Read the model definition and answer for the solid it produces. Units are mm, in the model's axes. A direction names the side the tool comes from. Coordinates: 2 decimals unless noted, no trailing zeros. Loops run counter-clockwise (first coordinate to the right, second up) from the corner with the lowest first, then second, coordinate; pieces in that order, holes last. Notation, with made-up numbers: (-25.75, 24) -> (-11.75, 24) arc R33 cw to (-11.75, 52) -> close; hole circle Ø2 at (43, -3). An arc over 180 degrees is marked (long way). Answer as a JSON object with one key per item and string values. Group by question number.
1) Section C-C, the plane x = 35.5 is taken. Give the vertices of the cut face in (y, z), plus the area to 3 significant figures.
2) Flat-ended cylindrical pins translate along their axes: P1, Ø0.7, axis at x = 14.5, y = -2, coming from the -Z side; P2, Ø1.5, axis at y = -2, z = -1, coming from the -X side; P3, Ø10, axis at x = 8.5, z = 47, coming from the +Y side; P4, Ø0.5, axis at x = 24.5, y = -1, coming from the +Z side. Find the tip coordinate at first contact, or state that the pin passes through.
3) Consider probe 1 along Z at (x, y) = (-2, -2.45); probe 2 along X at (y, z) = (-2.5, 113); probe 3 along Z at (x, y) = (46, -0.15). Determine where each line is inside the solid, lowest interval first. Write a range as [from, to].
4) Section A-A, the plane z = 91 is taken. Give the vertices of the cut face in (x, y).
5) Determine the mould class of faces 1 (the face through (-15.873, -1.503, 63.725)), 2 (the face through (41.28, -1.5, 0.14)), 3 (the face through (3, 0, 43)) for opening direction Z: released by +Z, released by -Z, zero draft, split by the parting line, or undercut.
6) Section B-B, the plane y = -2 is taken. Count the separate pieces of the cut face and the enclosed holes in it, plus the area to 3 significant figures.
7) Which of the six approach directions +Z, -Z, +X, -X, +Y, -Y give full straight-line access (tool end or side, diameter ignored) to faces 4 (the face through (21.838, -2, -2)), 5 (the face through (0.193, -1.503, 123.823)), 6 (the face through (13.537, -1.503, 39.443))?
from build123d import *

# Parameters (mm, degrees)
F0_R     = 3.175
F0_W     = 0.6713387143
F0_H     = 5.7765472419
F1_DEPTH = 3.048


with BuildPart() as f1:
    # F0 (on Front) → F1 (new body)
    with BuildSketch(Plane.XZ):
        with BuildLine():
            ThreePointArc((0.3401785714, -9.5189234444), (6.8544082857, -6.6138273378), (9.525, 0))
            ThreePointArc((9.525, 0), (-0.4768479324, 9.5130563464), (-9.4772553384, -0.9525))
            ThreePointArc((-9.4772553384, -0.9525), (-6.2623833816, -7.1769199091), (0.3401785714, -9.5189234444))
        make_face()
        Circle(F0_R, mode=Mode.SUBTRACT)
        with BuildLine():
            ThreePointArc((-9.4772553384, -0.9525), (-0.4768479324, 9.5130563464), (9.525, 0))
            ThreePointArc((9.525, 0), (6.8544082857, -6.6138273378), (0.3401785714, -9.5189234444))
            Line((0.3401785714, -9.5189234444), (44.7334821429, -7.9324362036))
            ThreePointArc((44.7334821429, -7.9324362036), (36.5125, 0), (44.7334821429, 7.9324362036))
            Line((44.7334821429, 7.9324362036), (18.9676000005, 8.8532337108))
            ThreePointArc((18.9676000005, 8.8532337108), (13.2611998974, 11.5713591498), (11.3411865923, 17.5933818124))
            Line((11.3411865923, 17.5933818124), (15.7954255641, 61.9125))
            ThreePointArc((15.7954255641, 61.9125), (0, 47.625), (-15.7954255641, 61.9125))
            Line((-15.7954255641, 61.9125), (-9.4772553384, -0.9525))
        make_face()
        with Locations((14.8607160592, -0.1777730082)):
            Rectangle(F0_W, F0_H, mode=Mode.SUBTRACT)
        with BuildLine():
            Line((19.8312775565, -3.0660466291), (19.3445253814, -3.0660466291))
            Line((19.3445253814, -3.0660466291), (19.2143033709, -2.4490724435))
            Line((19.2143033709, -2.4490724435), (19.1826960868, -2.4490724435))
            add(Edge.make_bspline(
                [(19.1826960868, -2.4490724435), (18.8590374977, -2.8561742627), (18.5372753455, -3.0009356239)],
                knots=[0, 0, 0, 1, 1, 1], degree=2))
            add(Edge.make_bspline(
                [(18.5372753455, -3.0009356239), (18.2155131934, -3.145696985), (17.7325538924, -3.145696985)],
                knots=[0, 0, 0, 1, 1, 1], degree=2))
            add(Edge.make_bspline(
                [(17.7325538924, -3.145696985), (17.0890295881, -3.145696985), (16.7236493839, -2.8131883563)],
                knots=[0, 0, 0, 1, 1, 1], degree=2))
            add(Edge.make_bspline(
                [(16.7236493839, -2.8131883563), (16.3582691798, -2.4806797276), (16.3582691798, -1.8687627074)],
                knots=[0, 0, 0, 1, 1, 1], degree=2))
            add(Edge.make_bspline(
                [(16.3582691798, -1.8687627074), (16.3582691798, -0.557692563), (18.4557285526, -0.4944779948)],
                knots=[0, 0, 0, 1, 1, 1], degree=2))
            Line((18.4557285526, -0.4944779948), (19.190281835, -0.4704564589))
            Line((19.190281835, -0.4704564589), (19.190281835, -0.2011623984))
            add(Edge.make_bspline(
                [(19.190281835, -0.2011623984), (19.190281835, 0.3083470213), (18.971559429, 0.5510909631)],
                knots=[0, 0, 0, 1, 1, 1], degree=2))
            add(Edge.make_bspline(
                [(18.971559429, 0.5510909631), (18.7528370231, 0.793834905), (18.2698777221, 0.793834905)],
                knots=[0, 0, 0, 1, 1, 1], degree=2))
            add(Edge.make_bspline(
                [(18.2698777221, 0.793834905), (17.7287610183, 0.793834905), (17.0460436818, 0.4625905677)],
                knots=[0, 0, 0, 1, 1, 1], degree=2))
            Line((17.0460436818, 0.4625905677), (16.8437570635, 0.9645142392))
            add(Edge.make_bspline(
                [(16.8437570635, 0.9645142392), (17.1636227786, 1.137722156), (17.5448066248, 1.2363368824)],
                knots=[0, 0, 0, 1, 1, 1], degree=2))
            add(Edge.make_bspline(
                [(17.5448066248, 1.2363368824), (17.9259904711, 1.3349516088), (18.3103350457, 1.3349516088)],
                knots=[0, 0, 0, 1, 1, 1], degree=2))
            add(Edge.make_bspline(
                [(18.3103350457, 1.3349516088), (19.0840813604, 1.3349516088), (19.4576794585, 0.9916965035)],
                knots=[0, 0, 0, 1, 1, 1], degree=2))
            add(Edge.make_bspline(
                [(19.4576794585, 0.9916965035), (19.8312775565, 0.6484413982), (19.8312775565, -0.1101334202)],
                knots=[0, 0, 0, 1, 1, 1], degree=2))
            Line((19.8312775565, -0.1101334202), (19.8312775565, -3.0660466291))
        make_face(mode=Mode.SUBTRACT)
        with BuildLine():
            Line((24.8012069082, -3.0660466291), (24.1450396903, -3.0660466291))
            Line((24.1450396903, -3.0660466291), (24.1450396903, -0.2643769666))
            add(Edge.make_bspline(
                [(24.1450396903, -0.2643769666), (24.1450396903, 0.2640968235), (23.9041921855, 0.5251729902)],
                knots=[0, 0, 0, 1, 1, 1], degree=2))
            add(Edge.make_bspline(
                [(23.9041921855, 0.5251729902), (23.6633446806, 0.7862491568), (23.1487780955, 0.7862491568)],
                knots=[0, 0, 0, 1, 1, 1], degree=2))
            add(Edge.make_bspline(
                [(23.1487780955, 0.7862491568), (22.4698536331, 0.7862491568), (22.1537807921, 0.4189725156)],
                knots=[0, 0, 0, 1, 1, 1], degree=2))
            add(Edge.make_bspline(
                [(22.1537807921, 0.4189725156), (21.8377079511, 0.0516958744), (21.8377079511, -0.7941150481)],
                knots=[0, 0, 0, 1, 1, 1], degree=2))
            Line((21.8377079511, -0.7941150481), (21.8377079511, -3.0660466291))
            Line((21.8377079511, -3.0660466291), (21.1815407332, -3.0660466291))
            Line((21.1815407332, -3.0660466291), (21.1815407332, 1.2641512924))
            Line((21.1815407332, 1.2641512924), (21.7150716888, 1.2641512924))
            Line((21.7150716888, 1.2641512924), (21.8212721634, 0.6711986427))
            Line((21.8212721634, 0.6711986427), (21.8528794475, 0.6711986427))
            add(Edge.make_bspline(
                [(21.8528794475, 0.6711986427), (22.0551660657, 0.9910643578), (22.4186498328, 1.1674330031)],
                knots=[0, 0, 0, 1, 1, 1], degree=2))
            add(Edge.make_bspline(
                [(22.4186498328, 1.1674330031), (22.7821336, 1.3438016483), (23.2284284515, 1.3438016483)],
                knots=[0, 0, 0, 1, 1, 1], degree=2))
            add(Edge.make_bspline(
                [(23.2284284515, 1.3438016483), (24.0110248057, 1.3438016483), (24.406115857, 0.9664106762)],
                knots=[0, 0, 0, 1, 1, 1], degree=2))
            add(Edge.make_bspline(
                [(24.406115857, 0.9664106762), (24.8012069082, 0.5890197041), (24.8012069082, -0.241619722)],
                knots=[0, 0, 0, 1, 1, 1], degree=2))
            Line((24.8012069082, -0.241619722), (24.8012069082, -3.0660466291))
        make_face(mode=Mode.SUBTRACT)
        with BuildLine():
            ThreePointArc((-15.7504882737, 65.484375), (-15.8737438155, 63.6997054867), (-15.7954255641, 61.9125))
            ThreePointArc((-15.7954255641, 61.9125), (0, 47.625), (15.7954255641, 61.9125))
            ThreePointArc((15.7954255641, 61.9125), (15.8550939106, 62.7052534459), (15.875, 63.5))
            ThreePointArc((15.875, 63.5), (15.8438414904, 64.4941387366), (15.7504882737, 65.484375))
            ThreePointArc((15.7504882737, 65.484375), (0, 79.375), (-15.7504882737, 65.484375))
        make_face()
        with Locations((0, 63.5)):
            Circle(F0_R, mode=Mode.SUBTRACT)
        with BuildLine():
            ThreePointArc((44.7334821429, 7.9324362036), (36.5125, 0), (44.7334821429, -7.9324362036))
            ThreePointArc((44.7334821429, -7.9324362036), (50.1620069047, -5.5115227815), (52.3875, 0))
            ThreePointArc((52.3875, 0), (50.1620069047, 5.5115227815), (44.7334821429, 7.9324362036))
        make_face()
        with Locations((44.45, 0)):
            Circle(F0_R, mode=Mode.SUBTRACT)
        with BuildLine():
            Line((-9.4502929642, 115.490625), (-15.7504882737, 65.484375))
            ThreePointArc((-15.7504882737, 65.484375), (0, 79.375), (15.7504882737, 65.484375))
            Line((15.7504882737, 65.484375), (9.4502929642, 115.490625))
            ThreePointArc((9.4502929642, 115.490625), (9.5063048942, 114.896483242), (9.525, 114.3))
            ThreePointArc((9.525, 114.3), (-0.596483242, 104.7936951058), (-9.4502929642, 115.490625))
        make_face()
        with Locations((-3.175, 100.0252)):
            Circle(F0_R, mode=Mode.SUBTRACT)
        with BuildLine():
            ThreePointArc((9.4502929642, 115.490625), (0, 123.825), (-9.4502929642, 115.490625))
            ThreePointArc((-9.4502929642, 115.490625), (-0.596483242, 104.7936951058), (9.525, 114.3))
            ThreePointArc((9.525, 114.3), (9.5063048942, 114.896483242), (9.4502929642, 115.490625))
        make_face()
        with Locations((0, 114.3)):
            Circle(F0_R, mode=Mode.SUBTRACT)
    extrude(amount=F1_DEPTH)


solid = f1.part
Determined:
{
 "1": {"outline": "(-3.05, -8.26) -> (0, -8.26) -> (0, 8.26) -> (-3.05, 8.26) -> close", "area": "50.4 mm²"},
 "2": {"P1": "z = -9.03", "P2": "x = -9.55", "P3": "y = 0", "P4": "z = 8.66"},
 "3": {"probe 1": "[-9.31, -2.47], [2.47, 61.03], [65.97, 97.08], [102.97, 111.83], [116.77, 123.61]", "probe 2": "[-9.76, -2.9], [2.9, 9.76]", "probe 3": "[-7.78, -2.77], [2.77, 7.78]"},
 "4": {"outline": "(-12.54, -3.05) -> (12.54, -3.05) -> (12.54, 0) -> (-12.54, 0) -> close"},
 "5": {"face 1": "split by the parting line", "face 2": "undercut", "face 3": "zero draft"},
 "6": {"separate pieces": "1", "enclosed holes": "8", "area": "3,750 mm²"},
 "7": {"face 4": "+Y, -Y", "face 5": "+Z, +Y, -Y", "face 6": "+X, +Y, -Y"}
}
